from build123d import *

# Parameters (mm, degrees)
BOX_W           = 50
BOX_H           = 90
BOX_DEPTH       = 3.1
SKETCH005_W     = 48
SKETCH005_H     = 100
PAD003_DEPTH    = 20
SKETCH006_W     = 42.1
SKETCH006_H     = 100
POCKET002_DEPTH = 16
SKETCH007_W     = 8.1
SKETCH007_H     = 100
POCKET003_DEPTH = 2
POCKET004_DEPTH = 100.001


with BuildPart() as cube:
    # Box → Box (new body)
    with BuildSketch(Plane(origin=(-25, -45, -10.55), x_dir=(1, 0, 0), z_dir=(0, 0, 1))):
        with Locations((25, 45)):
            Rectangle(BOX_W, BOX_H)
    extrude(amount=BOX_DEPTH)


with BuildPart() as base:
    # Sketch005 → Pad003 (new body)
    with BuildSketch(Plane.XY):
        Rectangle(SKETCH005_W, SKETCH005_H)
    extrude(amount=PAD003_DEPTH)

    # Sketch006 (on Face6 of Pad003) → Pocket002 (cut)
    with BuildSketch(Plane.XY.offset(20)):
        Rectangle(SKETCH006_W, SKETCH006_H)
    extrude(amount=-POCKET002_DEPTH, mode=Mode.SUBTRACT)

    # Sketch007 (on Face6 of Pocket002) → Pocket003 (cut)
    with BuildSketch(Plane.XY.offset(4)):
        with Locations((-14, 0)):
            Rectangle(SKETCH007_W, SKETCH007_H)
        with Locations((14, 0)):
            Rectangle(SKETCH007_W, SKETCH007_H)
    extrude(amount=-POCKET003_DEPTH, mode=Mode.SUBTRACT)

    # Sketch008 (on Face18 of Pocket003) → Pocket004 (cut, through all)
    with BuildSketch(Plane.XZ.offset(50)):
        Polygon((-18.05, 2), (-19.05, 2), (-18.05, 4), align=None)
        Polygon((-9.95, 2), (-8.95, 2), (-9.95, 4), align=None)
        Polygon((9.95, 2), (8.95, 2), (9.95, 4), align=None)
        Polygon((18.05, 2), (19.05, 2), (18.05, 4), align=None)
    extrude(amount=-POCKET004_DEPTH, mode=Mode.SUBTRACT)


with BuildPart() as base_1:
    # Body003 placement: moved
    add(base.part.moved(Location((0, 0, -25))))

    # Cut002: cut Cube
    add(cube.part, mode=Mode.SUBTRACT)


solid = base_1.part
Could you check a few things on this model? Use its own coordinates, in mm. A direction names the side the tool comes from. Round coordinates to 2 decimals unless told otherwise and drop trailing zeros. Order: outer loops, then holes, each group sorted by start corner. A loop starts at its lowest first (then second) coordinate and runs counter-clockwise, first axis right, second up.
(1) Imagine slicing it at D-D (x = -0.5). Write out the boundary of the cut face in (y, z), plus the area to 3 significant figures.
Response values:
outline: (-50, -25) - (50, -25) - (50, -21) - (-50, -21) - close
area: 400 mm2
(2) Imagine slicing it at B-B (z = -9). Write out the boundary of the cut face in (x, y).
Response values:
outline: (-24, -50) - (-21.05, -50) - (-21.05, -45) - (-24, -45) - close; (-24, 45) - (-21.05, 45) - (-21.05, 50) - (-24, 50) - close; (21.05, -50) - (24, -50) - (24, -45) - (21.05, -45) - close; (21.05, 45) - (24, 45) - (24, 50) - (21.05, 50) - close
(3) Imagine slicing it at C-C (x = -17). Write out the boundary of the cut face in (y, z), plus the area to 3 significant figures.
Response values:
outline: (-50, -25) - (50, -25) - (50, -23) - (-50, -23) - close
area: 200 mm2
(4) Please list where these lines run through material, in increasing order: line 1 along X through (y, z) = (18.5, -20); line 2 along X through (y, z) = (36.5, -22.25) (3 decimals); line 3 along Y through (x, z) = (21.5, -10).
Response values:
line 1: x = -24 to -21.05, 21.05 to 24
line 2: x = -24 to -18.675, -9.325 to 9.325, 18.675 to 24
line 3: y = -50 to -45, 45 to 50
(5) Which directions (+Z, -Z, +X, -X, +Y, -Y) give clear straight access to the entire face, cutting with the end or side of a thin tool? Please do faces 1 (the flat face through (20, 1, -21)), 2 (the flat face through (23, 1, -10.55)), 3 (the flat face through (14, -1, -23)), 4 (the flat face through (-24, -1, -15)).
Response values:
face 1: +Z, +Y, -Y
face 2: +X, -X
face 3: +Y, -Y
face 4: +Z, -Z, -X, +Y, -Y
(6) Imagine slicing it at A-A (y = -26). Write out the boundary of the cut face in (x, z), plus the area to 3 significant figures.
Response values:
outline: (-24, -25) - (24, -25) - (24, -10.55) - (21.05, -10.55) - (21.05, -21) - (18.05, -21) - (19.05, -23) - (8.95, -23) - (9.95, -21) - (-9.95, -21) - (-8.95, -23) - (-19.05, -23) - (-18.05, -21) - (-21.05, -21) - (-21.05, -10.55) - (-24, -10.55) - close; (-24, -7.45) - (-21.05, -7.45) - (-21.05, -5) - (-24, -5) - close; (21.05, -7.45) - (24, -7.45) - (24, -5) - (21.05, -5) - close
area: 232 mm2
(7) I'm going to push flat-ended pins straight in: pin 1 (5 mm diameter, centred on x = 2, y = 24, fed in from +Z); pin 2 (1.5 mm diameter, centred on x = 11, y = 6, fed in from +Z). Where does each tip first touch, or does it pass through?
Response values:
pin 1: stops at z = -21
pin 2: stops at z = -23
(8) If we mould it in two halves opening along Y, with no side actions, what happens to faces 5 (the flat face through (23, 1, -7.45)), 6 (the flat face through (-14, -1, -23))? For each: released by +Y, released by -Y, zero draft, split by the parting line, or undercut.
Response values:
face 5: undercut
face 6: zero draft
